```python
from build123d import *

# Parameters (mm, degrees)
SKETCH_1_W          = 5.6
SKETCH_1_H          = 65
SKETCH_2_R          = 25
CUT_EXTRUDE_1_DEPTH = 93.094299498
SKETCH_3_R          = 2.1
CUT_EXTRUDE_2_DEPTH = 93.094299498


with BuildPart() as part:
    # ｽｹｯﾁ1 → 回転1 (revolve)
    with BuildSketch(Plane(origin=(0, 0, 0), x_dir=(0, 0, -1), z_dir=(1, 0, 0))):
        with Locations((-2.8, 32.5)):
            Rectangle(SKETCH_1_W, SKETCH_1_H)
    revolve(axis=Axis((0, 0, 0), (0, 0, 1)))

    # ｽｹｯﾁ2 → ｶｯﾄ - 押し出し1 (cut, through all)
    with BuildSketch(Plane(origin=(0, 0, 0), x_dir=(-1, 0, 0), z_dir=(0, 0, -1))):
        with Locations(Location((0, 0, 0), (0, 0, 90))):
            Circle(SKETCH_2_R)
    extrude(amount=-CUT_EXTRUDE_1_DEPTH, mode=Mode.SUBTRACT)

    # ｽｹｯﾁ3 → ｶｯﾄ - 押し出し2 (cut, through all)
    with BuildSketch(Plane(origin=(0, 0, 0), x_dir=(-1, 0, 0), z_dir=(0, 0, -1))):
        with Locations(Location((0, 44.45, 0), (0, 0, 90))):
            Circle(SKETCH_3_R)
        with Locations(Location((44.45, 0, 0), (0, 0, 90))):
            Circle(SKETCH_3_R)
        with Locations(Location((0, -44.45, 0), (0, 0, 90))):
            Circle(SKETCH_3_R)
        with Locations(Location((-44.45, 0, 0), (0, 0, 90))):
            Circle(SKETCH_3_R)
    extrude(amount=-CUT_EXTRUDE_2_DEPTH, mode=Mode.SUBTRACT)


solid = part.part
```
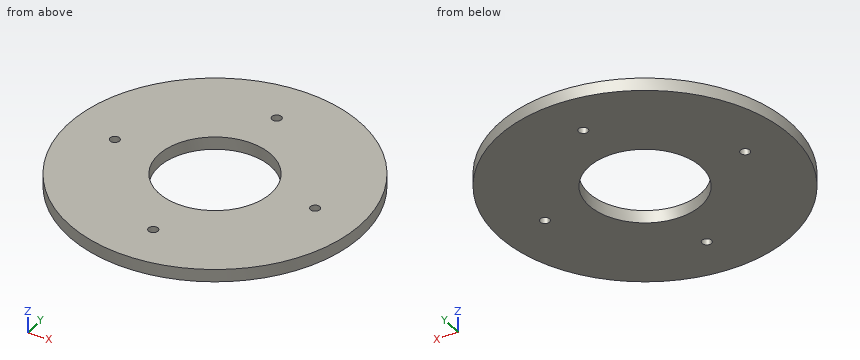
CAD build for the part. Positions are in the model's coordinates, mm. Coordinates: 2 decimals unless noted, no trailing zeros. Write each loop counter-clockwise with the first axis right and the second up, starting at its lowest first coordinate (ties: lowest second). Pieces come first, ordered by that corner, then holes. Notation, with made-up numbers: (56, 33) -> (66, 33) arc R27 ccw to (66, 51) -> close; hole circle Ø2 at (64, -40). An arc over 180 degrees is marked (long way). Use CSV: the item, a comma, the result in double quotes. Start each with the question number.
Item 1: Wall check: probe 1 along X at (y, z) = (0, 4.2); probe 2 along Y at (x, z) = (-15, 5.1); probe 3 along X at (y, z) = (44.45, 2.4). Give the ranges that are in metal, low to high.
Item 2: Band-saw the part on C-C, the plane z = 1.75. Write the cut outline in (x, y).
Item 3: Band-saw the part on A-A, the plane y = 0. Write the cut outline in (x, z), plus the area to 3 significant figures.
Item 4: Band-saw the part on D-D, the plane y = -45. Write the cut outline in (x, z).
Item 5: Drop flat-ended pins along their axis: P1, Ø1.5, axis at y = -22, z = 2.5, coming from the +X side; P2, Ø2.5, axis at x = -44.45, y = 0, coming from the -Z side; P3, Ø2, axis at x = 6, z = 4, coming from the +Y side; P4, Ø1, axis at x = 40.5, z = 3, coming from the +Y side. Give the stop position or say it passes through.
Response values:
1,probe 1,"x = -65 to -46.55, -42.35 to -25, 25 to 42.35, 46.55 to 65"
1,probe 2,"y = -63.25 to -20, 20 to 63.25"
1,probe 3,"x = -47.43 to -2.1, 2.1 to 47.43"
2,outline,"circle Ø130 at (0, 0); hole circle Ø4.2 at (-44.45, 0); hole circle Ø50 at (0, 0); hole circle Ø4.2 at (0, -44.45); hole circle Ø4.2 at (0, 44.45); hole circle Ø4.2 at (44.45, 0)"
3,outline,"(-65, 0) -> (-46.55, 0) -> (-46.55, 5.6) -> (-65, 5.6) -> close; (-42.35, 0) -> (-25, 0) -> (-25, 5.6) -> (-42.35, 5.6) -> close; (25, 0) -> (42.35, 0) -> (42.35, 5.6) -> (25, 5.6) -> close; (46.55, 0) -> (65, 0) -> (65, 5.6) -> (46.55, 5.6) -> close"
3,area,"401 mm2"
4,outline,"(-46.9, 0) -> (-2.03, 0) -> (-2.03, 5.6) -> (-46.9, 5.6) -> close; (2.03, 0) -> (46.9, 0) -> (46.9, 5.6) -> (2.03, 5.6) -> close"
5,P1,"stops at x = 61.43"
5,P2,"passes through"
5,P3,"stops at y = 64.81"
5,P4,"stops at y = 51.23"
